```python
from build123d import *

# Parameters (mm, degrees)
CROQUIS1_W              = 131.9512
CROQUIS1_H              = 130.6
CROQUIS1_W_2            = 42.2512
CROQUIS1_H_2            = 105.2
CROQUIS1_W_3            = 51.6
CROQUIS1_H_3            = 46.25
SALIENTE_EXTRUIR1_DEPTH = 12.7
CROQUIS2_W              = 12.7
CROQUIS2_H              = 12.7
SALIENTE_EXTRUIR2_DEPTH = 158
CROQUIS3_W              = 131.9512
CROQUIS3_H              = 130.6
CROQUIS3_W_2            = 106.5512
CROQUIS3_H_2            = 105.2
SALIENTE_EXTRUIR3_DEPTH = 12.7
SALIENTE_EXTRUIR4_REACH = 256.78
CROQUIS4_W              = 12.7
CROQUIS4_H              = 12.7
SALIENTE_EXTRUIR5_DEPTH = 12.7


with BuildPart() as part:
    # Croquis1 → Saliente-Extruir1 (new body)
    with BuildSketch(Plane(origin=(0, 0, 0), x_dir=(1, 0, 0), z_dir=(0, 1, 0))):
        with Locations((65.9756, 65.3)):
            Rectangle(CROQUIS1_W, CROQUIS1_H)
        with Locations((33.8256, 65.3)):
            Rectangle(CROQUIS1_W_2, CROQUIS1_H_2, mode=Mode.SUBTRACT)
        with Locations((93.4512, 35.825)):
            Rectangle(CROQUIS1_W_3, CROQUIS1_H_3, mode=Mode.SUBTRACT)
        with Locations((93.4512, 94.775)):
            Rectangle(CROQUIS1_W_3, CROQUIS1_H_3, mode=Mode.SUBTRACT)
    extrude(amount=SALIENTE_EXTRUIR1_DEPTH)

    # Croquis2 → Saliente-Extruir2 (add)
    with BuildSketch(Plane(origin=(0, 12.7, 0), x_dir=(1, 0, 0), z_dir=(0, 1, 0))):
        with Locations((6.35, 124.25)):
            Rectangle(CROQUIS2_W, CROQUIS2_H)
        with Locations((6.35, 6.35)):
            Rectangle(CROQUIS2_W, CROQUIS2_H)
        with Locations((125.6012, 124.25)):
            Rectangle(CROQUIS2_W, CROQUIS2_H)
        with Locations((125.6012, 6.35)):
            Rectangle(CROQUIS2_W, CROQUIS2_H)
    extrude(amount=SALIENTE_EXTRUIR2_DEPTH)

    # Croquis3 → Saliente-Extruir3 (add)
    with BuildSketch(Plane(origin=(0, 170.7, 0), x_dir=(1, 0, 0), z_dir=(0, 1, 0))):
        with Locations((65.9756, 65.3)):
            Rectangle(CROQUIS3_W, CROQUIS3_H)
        with Locations((65.9756, 65.3)):
            Rectangle(CROQUIS3_W_2, CROQUIS3_H_2, mode=Mode.SUBTRACT)
    extrude(amount=SALIENTE_EXTRUIR3_DEPTH)

    # Croquis4 → Saliente-Extruir4 (add, up to next)
    with BuildSketch(Plane.ZY.offset(-119.2512), mode=Mode.PRIVATE) as saliente_extruir4_sk1:
        with Locations((-6.35, 119.05)):
            Rectangle(CROQUIS4_W, CROQUIS4_H)
    saliente_extruir4_tool1 = extrude(saliente_extruir4_sk1.sketch, amount=SALIENTE_EXTRUIR4_REACH, mode=Mode.PRIVATE) - part.part
    # Croquis4 → Saliente-Extruir4 (add, up to next)
    with BuildSketch(Plane.ZY.offset(-119.2512), mode=Mode.PRIVATE) as saliente_extruir4_sk2:
        with Locations((-124.25, 119.05)):
            Rectangle(CROQUIS4_W, CROQUIS4_H)
    saliente_extruir4_tool2 = extrude(saliente_extruir4_sk2.sketch, amount=SALIENTE_EXTRUIR4_REACH, mode=Mode.PRIVATE) - part.part
    add(saliente_extruir4_tool1.solids().sort_by_distance((119.2512, 119.05, -6.35))[0])
    add(saliente_extruir4_tool2.solids().sort_by_distance((119.2512, 119.05, -124.25))[0])

    # Croquis5 → Saliente-Extruir5 (add)
    with BuildSketch(Plane(origin=(0, 12.7, 0), x_dir=(1, 0, 0), z_dir=(0, 1, 0))):
        Polygon((131.9512, 96.3), (154.9512, 96.3), (154.9512, 34.3), (131.9512, 34.3), (131.9512, 40.3), (148.9512, 40.3), (148.9512, 90.3), (131.9512, 90.3), align=None)
    extrude(amount=-SALIENTE_EXTRUIR5_DEPTH)


solid = part.part
```
For this review, take the finished solid that the model builds, in its own axes (mm). A direction names the side the tool comes from. Coordinates: 2 decimals unless noted, no trailing zeros. Write each loop counter-clockwise with the first axis right and the second up, starting at its lowest first coordinate (ties: lowest second). Pieces come first, ordered by that corner, then holes.
(1) Add section C-C on x = 35. Give the boundary of the cut face in (y, z).
(2) Add section D-D on y = 68. Give the boundary of the cut face in (x, z).
(3) Tool access review of faces 4 (the face through (6, 12.7, -66)), 5 (the face through (12.7, 6, -65)), 6 (the face through (12.7, 62, -6)), 7 (the face through (143, 6, -96.3)): name each direction out of +Z, -Z, +X, -X, +Y, -Y from which nothing blocks a thin tool from reaching the whole face with its end or side.
(4) Wall thickness on probe 1 along X at (y, z) = (9, -89); probe 2 along Y at (x, z) = (88, -6.5); probe 3 along X at (y, z) = (66.5, -8): over which ranges is each line inside the solid? List them lowest first.
(5) For pin 1 Ø4 at (x, z) = (139, -39.5) entering from -Y; pin 2 Ø10 at (y, z) = (77.5, -4) entering from +X; pin 3 Ø6.5 at (x, y) = (139.5, 5.5) entering from -Z; pin 4 Ø8 at (x, z) = (91, -65.5) entering from +Y, all flat-tipped, find the tip position at first contact; note any pin that passes through.
(6) Add section A-A on x = 144. Give the boundary of the cut face in (y, z), then the cut area to 3 significant figures.
(7) Add section B-B on z = -23. Give the boundary of the cut face in (x, y).
(8) The part is to be moulded in two halves that separate along Y. For faces 1 (the face through (93, 6, -71.65)), 2 (the face through (65, 183.4, -8)), 3 (the face through (119.251, 62, -6)), say which applies: +Y half, -Y half, draft (parallel to the pull), parting line (faces both ways), or undercut.
Answer sheet:
1. outline: (0, -130.6) - (12.7, -130.6) - (12.7, -117.9) - (0, -117.9) - close; (0, -12.7) - (12.7, -12.7) - (12.7, 0) - (0, 0) - close; (112.7, -130.6) - (125.4, -130.6) - (125.4, -117.9) - (112.7, -117.9) - close; (112.7, -12.7) - (125.4, -12.7) - (125.4, 0) - (112.7, 0) - close; (170.7, -130.6) - (183.4, -130.6) - (183.4, -117.9) - (170.7, -117.9) - close; (170.7, -12.7) - (183.4, -12.7) - (183.4, 0) - (170.7, 0) - close
2. outline: (0, -130.6) - (12.7, -130.6) - (12.7, -117.9) - (0, -117.9) - close; (0, -12.7) - (12.7, -12.7) - (12.7, 0) - (0, 0) - close; (119.25, -130.6) - (131.95, -130.6) - (131.95, -117.9) - (119.25, -117.9) - close; (119.25, -12.7) - (131.95, -12.7) - (131.95, 0) - (119.25, 0) - close
3. face 4: +X, -X
3. face 5: +Y, -Y
3. face 6: +Z, -Z
3. face 7: -Z, +X, +Y, -Y
4. probe 1: x = 0 to 12.7, 54.95 to 67.65, 119.25 to 131.95, 148.95 to 154.95
4. probe 2: y = 0 to 12.7, 112.7 to 125.4, 170.7 to 183.4
4. probe 3: x = 0 to 12.7, 119.25 to 131.95
5. pin 1: stops at y = 0
5. pin 2: stops at x = 131.95
5. pin 3: stops at z = -96.3
5. pin 4: stops at y = 12.7
6. outline: (0, -96.3) - (12.7, -96.3) - (12.7, -90.3) - (0, -90.3) - close; (0, -40.3) - (12.7, -40.3) - (12.7, -34.3) - (0, -34.3) - close
6. area: 152 mm2
7. outline: (0, 0) - (12.7, 0) - (12.7, 12.7) - (0, 12.7) - close; (0, 170.7) - (12.7, 170.7) - (12.7, 183.4) - (0, 183.4) - close; (54.95, 0) - (67.65, 0) - (67.65, 12.7) - (54.95, 12.7) - close; (119.25, 0) - (131.95, 0) - (131.95, 12.7) - (119.25, 12.7) - close; (119.25, 170.7) - (131.95, 170.7) - (131.95, 183.4) - (119.25, 183.4) - close
8. face 1: draft
8. face 2: +Y half
8. face 3: undercut
